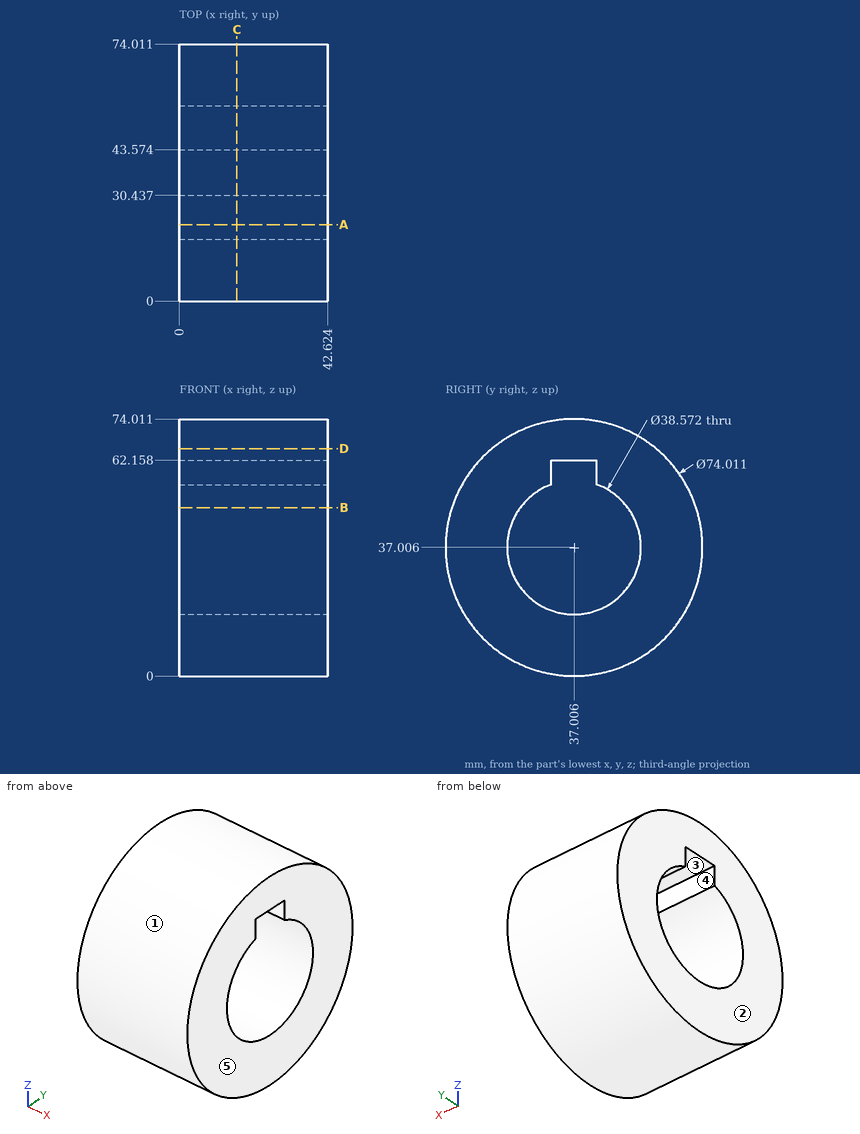
Geometry check sheet. Reference: drawing and pictorial views, mm from the part's lowest x, y, z. A direction names the side the tool comes from. Round coordinates to 2 decimals unless told otherwise and drop trailing zeros. Loops run counter-clockwise (first coordinate to the right, second up) from the corner with the lowest first, then second, coordinate; pieces in that order, holes last. Notation, with made-up numbers: (-16, 85.25) - (31, 85.25) arc R35 ccw to (31, 123.25) - close; hole circle Ø2 at (-11.75, 73.5). An arc over 180 degrees is marked (long way). Answer in a Markdown table with one row per item. Add a question column.
Q1. Release check for a two-part mould opening along Y. For the marked faces 1, 2 and 3 record: pulls with the +Y half, pulls with the -Y half, needs draft (parallel to the pull), parting line crosses it, or undercut.
Q2. Section check B-B on z = 48.5. Enter the section's corners in (x, y) (1 decimal), plus the area to 3 significant figures.
Q3. Section check A-A on y = 22. Enter the section's corners in (x, z) (1 decimal).
Q4. Material ranges on line 1 (Y direction, x = 5.5, z = 38) (1 decimal); line 2 (Z direction, x = 28.5, y = 46.5); line 3 (Z direction, x = 37, y = 30) (1 decimal), recorded low to high.
Q5. Section check D-D on z = 65.5. Enter the section's corners in (x, y) (1 decimal).
Q6. Section check C-C on x = 16.5. Enter the section's corners in (y, z) (1 decimal).
Q7. Gauge pin test, flat ends, axial feed: pin 1 (2 mm diameter, centred on x = 29, z = 11.5, fed in from +Y) (1 decimal); pin 2 (1.5 mm diameter, centred on x = 21.5, y = 17.5, fed in from -Z) (1 decimal); pin 3 (4 mm diameter, centred on x = 31.5, z = 58, fed in from -Y). Record the tip position at first contact, or that the pin passes through.
Q8. Tool access check on the marked faces 4 and 5. Record the directions out of +Z, -Z, +X, -X, +Y, -Y that give a thin tool (end or side, any length) a straight path to the whole face; none if there is none.
Found:
| question | item | result |
|---|---|---|
| 1 | face 1 | parting line crosses it |
| 1 | face 2 | needs draft |
| 1 | face 3 | undercut |
| 2 | outline | (0, 1.8) - (42.6, 1.8) - (42.6, 21.5) - (0, 21.5) - close; (0, 52.5) - (42.6, 52.5) - (42.6, 72.2) - (0, 72.2) - close |
| 2 | area | 1,680 mm² |
| 3 | outline | (0, 3.2) - (42.6, 3.2) - (42.6, 24.9) - (0, 24.9) - close; (0, 49.1) - (42.6, 49.1) - (42.6, 70.8) - (0, 70.8) - close |
| 4 | line 1 | y = 0 to 17.7, 56.3 to 74 |
| 4 | line 2 | z = 1.24 to 20.22, 53.79 to 72.77 |
| 4 | line 3 | z = 0.7 to 19, 55 to 73.3 |
| 5 | outline | (0, 13.4) - (42.6, 13.4) - (42.6, 60.6) - (0, 60.6) - close |
| 6 | outline | circle Ø74 at (37, 37); hole (30.4, 55.1) arc R19.3 ccw (long way) to (43.6, 55.1) - (43.6, 62.2) - (30.4, 62.2) - close |
| 7 | pin 1 | stops at y = 64.7 |
| 7 | pin 2 | stops at z = 5.1 |
| 7 | pin 3 | stops at y = 5.25 |
| 8 | face 4 | +X, -X |
| 8 | face 5 | +Z, -Z, +X, +Y, -Y |
